The drawing under review shows one solid part. Ordinate dimensions are in mm from its lowest x, y, z. Coordinates: 2 decimals unless noted, no trailing zeros. Write each loop counter-clockwise with the first axis right and the second up, starting at its lowest first coordinate (ties: lowest second). Pieces come first, ordered by that corner, then holes.
Q1. Take a section at B-B (x = 4.5). Give the boundary of the cut face in (y, z), and give its area (3 significant figures).
Q2. For probe 1 along Y at (x, z) = (3.5, 1) (1 decimal); probe 2 along X at (y, z) = (35, 3); probe 3 along X at (y, z) = (5, 2), list the stretches that pass through material, from the lowest coordinate up.
Q3. Take a section at A-A (z = 2.5). Give the boundary of the cut face in (x, y).
Q4. Mouldability with a two-part tool opening along Z and no side actions: class the marked faces 1, 2 and 3 as pulls with the +Z half, pulls with the -Z half, needs draft (parallel to the pull), parting line crosses it, or undercut.
Q5. Take a section at C-C (y = 12.5). Give the boundary of the cut face in (x, z), and give its area (3 significant figures).
Q6. Insertion check: pin 1 (2 mm diameter, centred on y = 14, z = 1.5, fed in from +X); pin 2 (2 mm diameter, centred on x = 31, y = 56, fed in from -Z). Each pin has a flat end and moves straight along its axis. Give the tip position at first contact, or say it passes through.
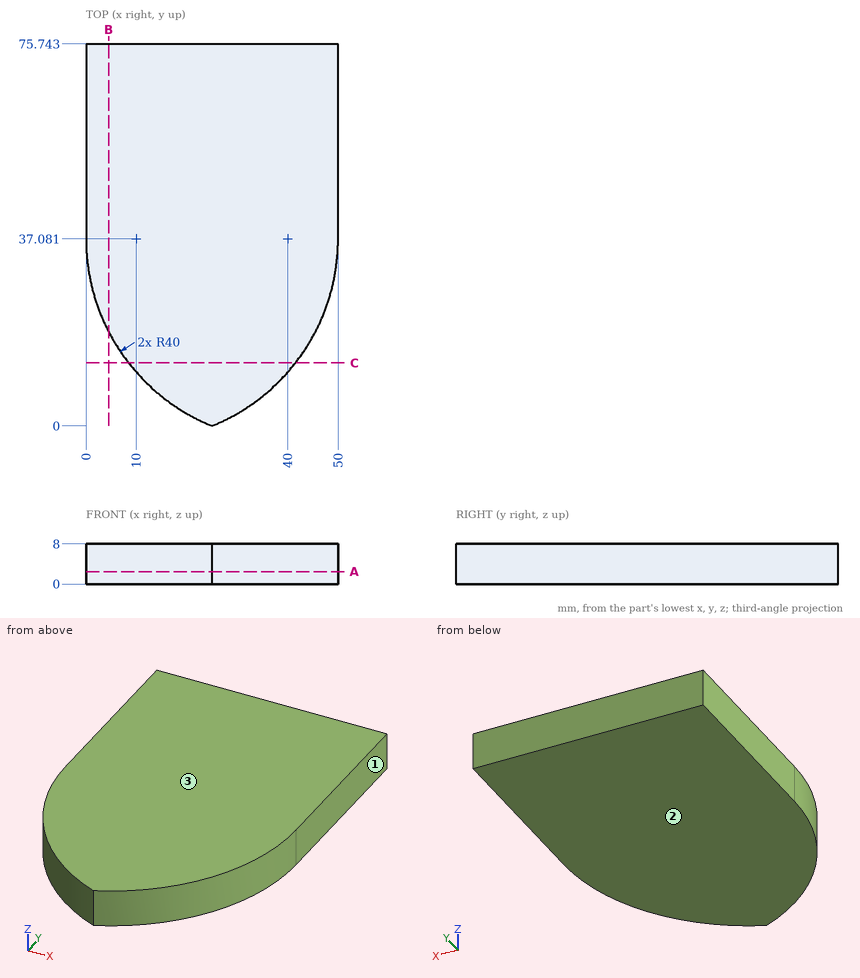
Response:
1. outline: (18.65, 0) - (75.74, 0) - (75.74, 8) - (18.65, 8) - close
1. area: 457 mm2
2. probe 1: y = 20.7 to 75.7
2. probe 2: x = 0.05 to 49.95
2. probe 3: x = 16.11 to 33.89
3. outline: (0, 37.08) arc R40 ccw to (25, 0) arc R40 ccw to (50, 37.08) - (50, 75.74) - (0, 75.74) - close
4. face 1: needs draft
4. face 2: pulls with the -Z half
4. face 3: pulls with the +Z half
5. outline: (8.44, 0) - (41.56, 0) - (41.56, 8) - (8.44, 8) - close
5. area: 265 mm2
6. pin 1: stops at x = 43.35
6. pin 2: stops at z = 0
